Verification items for this drawing (mm, ordinates from the low corner). Round coordinates to 2 decimals unless told otherwise and drop trailing zeros. Write each loop counter-clockwise with the first axis right and the second up, starting at its lowest first coordinate (ties: lowest second). Pieces come first, ordered by that corner, then holes. Notation, with made-up numbers: (50.5, 3.25) -> (67.5, 3.25) arc R16 cw to (67.5, 29.25) -> close; hole circle Ø6 at (66, 81.5). An arc over 180 degrees is marked (long way). Put each result on its own line as item: value. Start each with the question number.
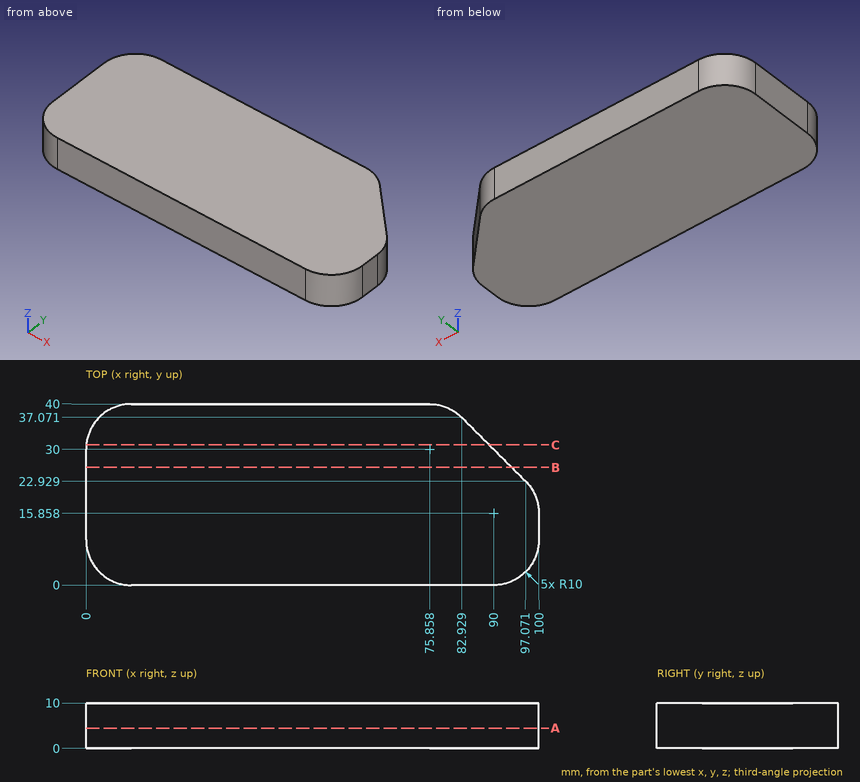
(1) Go/stop test with a flat-tipped pin: pin 1 Ø1 at (y, z) = (23, 5) entering from +X (1 decimal). Record where the tip stops, or that it passes through.
(2) Sectioned sample at B-B (y = 26). Record the cut outline in (x, z), and give its area (3 significant figures).
(3) Sectioned sample at A-A (z = 4.5). Record the cut outline in (x, y).
(4) Sectioned sample at C-C (y = 31). Record the cut outline in (x, z).
(5) Material ranges on L1, parallel to Y at x = 93, z = 5.5; L2, parallel to Y at x = 88.5, z = 5.75; L3, parallel to X at y = 34, z = 9.5 (1 decimal), recorded low to high. Write a range as from..to.
Found:
1. pin 1: x = 97.5
2. outline: (0, 0) -> (94, 0) -> (94, 10) -> (0, 10) -> close
2. area: 940 mm2
3. outline: (0, 10) arc R10 ccw to (10, 0) -> (90, 0) arc R10 ccw to (100, 10) -> (100, 15.86) arc R10 ccw to (97.07, 22.93) -> (82.93, 37.07) arc R10 ccw to (75.86, 40) -> (10, 40) arc R10 ccw to (0, 30) -> close
4. outline: (0.05, 0) -> (89, 0) -> (89, 10) -> (0.05, 10) -> close
5. L1: 0.46..27
5. L2: 0..31.5
5. L3: 0.8..86
